Source: CAD feature listing. Evaluate the final solid. Frame: model axes, mm. Round coordinates to 2 decimals unless told otherwise and drop trailing zeros. Write each loop counter-clockwise with the first axis right and the second up, starting at its lowest first coordinate (ties: lowest second). Pieces come first, ordered by that corner, then holes. Notation, with made-up numbers: M 76.25,6 L 90.25,6 A24 ccw 90.25,32 Z; hole C 69.25,14.5 d1. An arc over 180 degrees is marked long. Answer in a Markdown table with one row per item. Add a question column.
Item 1: Contact query for a flat-ended pin moving along its axis: pin 1 (1.9 mm diameter, centred on x = 5, y = 0, fed in from +Z). Output: stop coordinate, or through.
Item 2: Mould query, pull axis X, two halves, no side actions, for faces 1 (the face through (104.6, -0.09, 1.52)), 2 (the face through (-2, 0, 0)). Classes: released by +X, released by -X, zero draft, split by the parting line, or undercut.
Item 3: Material intervals for probe 1 along Y at (x, z) = (117.5, 1.05); probe 2 along Y at (x, z) = (5, 0.75), sorted ascending.
Item 4: Cut plane A-A on x = 102.5. Return loops of the section in (y, z), and give its area (3 significant figures).
from build123d import *

# Parameters (mm, degrees)
SKETCH_1_W          = 250
SKETCH_1_H          = 20
EXTRUDE_1_DEPTH     = 3
SKETCH_2_R          = 2.1
SKETCH_2_R_2        = 1.6
CUT_EXTRUDE_1_DEPTH = 3
FILLET_1_R          = 2


with BuildPart() as part:
    # 草图1 → 凸台-拉伸1 (new body)
    with BuildSketch(Plane.XY):
        Rectangle(SKETCH_1_W, SKETCH_1_H)
    extrude(amount=EXTRUDE_1_DEPTH)

    # 草图2 → 切除-拉伸1 (cut)
    with BuildSketch(Plane.XY.offset(3)):
        with Locations((-117.5, 0)):
            Circle(SKETCH_2_R)
        with Locations((-102.5, 0)):
            Circle(SKETCH_2_R)
        with Locations(Location((102.5, 0, 0), (0, 0, 180))):
            Circle(SKETCH_2_R)
        with Locations(Location((117.5, 0, 0), (0, 0, 180))):
            Circle(SKETCH_2_R)
        with Locations((-5, 0)):
            Circle(SKETCH_2_R_2)
        with Locations(Location((5, 0, 0), (0, 0, 180))):
            Circle(SKETCH_2_R_2)
    extrude(amount=-CUT_EXTRUDE_1_DEPTH, mode=Mode.SUBTRACT)

    # 圆角1
    fillet_1_edges = [part.edges().sort_by_distance(p)[0] for p in [
        (125, -10, 1.5),
        (-125, -10, 1.5),
        (-125, 10, 1.5),
        (125, 10, 1.5),
    ]]
    fillet(fillet_1_edges, radius=FILLET_1_R)


solid = part.part
Results below:
| question | item | result |
|---|---|---|
| 1 | pin 1 | through |
| 2 | face 1 | undercut |
| 2 | face 2 | zero draft |
| 3 | probe 1 | -10 to -2.1, 2.1 to 10 |
| 3 | probe 2 | -10 to -1.6, 1.6 to 10 |
| 4 | outline | M -10,0 L -2.1,0 L -2.1,3 L -10,3 Z; M 2.1,0 L 10,0 L 10,3 L 2.1,3 Z |
| 4 | area | 47.4 mm2 |
